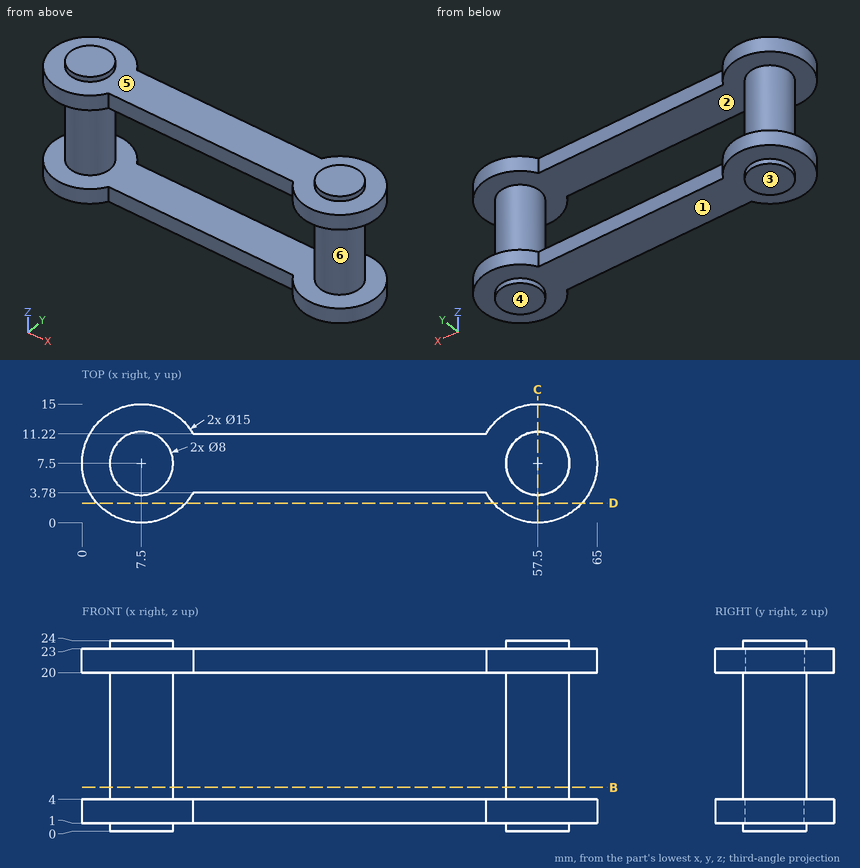
Design review of the part shown in the three views and the two pictorial views. Dimensions are in mm from the part's minimum x, y and z. A direction names the side the tool comes from. Give positions to 0.01 mm unless a question says otherwise; leave off trailing zeros. Order: outer loops, then holes, each group sorted by start corner. A loop starts at its lowest first (then second) coordinate and runs counter-clockwise, first axis right, second up. Notation, with made-up numbers: (79.25, 22) -> (114.25, 22) arc R13 cw to (114.25, 45) -> close; hole circle Ø10 at (-24, 48.5). An arc over 180 degrees is marked (long way). Write each question's results on one line, items separated by ' | '. Start each with the question number.
Q1. Add section D-D on y = 2.5. Give the boundary of the cut face in (x, z).
Q2. For pin 1 (3 mm diameter, centred on y = 10.5, z = 18, fed in from -X); pin 2 (8 mm diameter, centred on y = 4.5, z = 15.5, fed in from -X); pin 3 (2 mm diameter, centred on y = 11.5, z = 9.5, fed in from +X) (1 decimal); pin 4 (2 mm diameter, centred on x = 13.5, z = 13.5, fed in from -Y), all flat-tipped, find the tip position at first contact; note any pin that passes through.
Q3. Add section B-B on z = 5.5. Give the boundary of the cut face in (x, y).
Q4. Machinability: for the marked faces 1, 2 and 3, which of the approach directions +Z, -Z, +X, -X, +Y, -Y give a long, thin tool a straight path to every point of the face, cutting with its end or side? Answer none if there is none.
Q5. Add section C-C on x = 57.5. Give the boundary of the cut face in (y, z).
Q6. Wall thickness on L1, parallel to Z at x = 32, y = 9.75; L2, parallel to Y at x = 20, z = 2.5; L3, parallel to X at y = 7.5, z = 11.25: over which ranges is each line inside the solid? List them lowest first. Write a range as from..to.
Q7. Mouldability with a two-part tool opening along Z and no side actions: class the marked faces 4, 5 and 6 as +Z half, -Z half, draft (parallel to the pull), parting line (faces both ways), or undercut.
Found:
1) outline: (1.91, 1) -> (13.09, 1) -> (13.09, 4) -> (1.91, 4) -> close; (1.91, 20) -> (13.09, 20) -> (13.09, 23) -> (1.91, 23) -> close; (51.91, 1) -> (63.09, 1) -> (63.09, 4) -> (51.91, 4) -> close; (51.91, 20) -> (63.09, 20) -> (63.09, 23) -> (51.91, 23) -> close
2) pin 1: stops at x = 3.79 | pin 2: stops at x = 3.5 | pin 3: stops at x = 60.1 | pin 4: passes through
3) outline: circle Ø8 at (7.5, 7.5); circle Ø8 at (57.5, 7.5)
4) face 1: -Z | face 2: none | face 3: -Z, +X, -X, +Y, -Y
5) outline: (0, 1) -> (3.5, 1) -> (3.5, 0) -> (11.5, 0) -> (11.5, 1) -> (15, 1) -> (15, 4) -> (11.5, 4) -> (11.5, 20) -> (15, 20) -> (15, 23) -> (11.5, 23) -> (11.5, 24) -> (3.5, 24) -> (3.5, 23) -> (0, 23) -> (0, 20) -> (3.5, 20) -> (3.5, 4) -> (0, 4) -> close
6) L1: z = 1..4, 20..23 | L2: y = 3.78..11.22 | L3: x = 3.5..11.5, 53.5..61.5
7) face 4: -Z half | face 5: +Z half | face 6: undercut
